Design review of the part built by this model. Coordinates are the model's own, in mm. A direction names the side the tool comes from. Coordinates: 2 decimals unless noted, no trailing zeros. Loops run counter-clockwise (first coordinate to the right, second up) from the corner with the lowest first, then second, coordinate; pieces in that order, holes last. Notation, with made-up numbers: (27, -6.5) -> (52, -6.5) arc R21 cw to (52, 5.5) -> close; hole circle Ø5 at (84, 57). An arc over 180 degrees is marked (long way). Use a Markdown table: item, result. Add a question column.
Q1. For probe 1 along Y at (x, z) = (0, 7); probe 2 along Y at (x, z) = (0, 2); probe 3 along X at (y, z) = (8, 31), list the stretches that pass through material, from the lowest coordinate up.
Q2. Take a section at B-B on y = 5.5. Write out the cut boundary in (x, z) (3 decimals), plus the area to 3 significant figures.
Q3. Clearance check with flat-ended pins moving along their axes: pin 1 Ø0.9 at (x, z) = (-17, 30.5) entering from -Y; pin 2 Ø5 at (x, z) = (3.5, 25) entering from -Y; pin 3 Ø10 at (x, y) = (-5, 1) entering from +Z. State where each tip first meets the part, or that it passes through.
Q4. Take a section at D-D on x = -17. Write out the cut boundary in (y, z) (3 decimals), plus the area to 3 significant figures.
Q5. For faces 1 (the face through (17, -1.016, 27)), 2 (the face through (17, -8.382, 27)), 3 (the face through (-3, -8, 5.398)), list the 3-axis set-ups (+Z, -Z, +X, -X, +Y, -Y) from which the entire face can be reached by the end or side of a thin tool; tool diameter is ignored.
Q6. Draft analysis for pull direction Y (two halves, no side actions). For faces 4 (the face through (15.249, -5, 27)), 5 (the face through (-19.431, 7, 27)), 6 (the face through (-17, -8.382, 27)), state which applies: pulls with the +Y half, pulls with the -Y half, needs draft (parallel to the pull), parting line crosses it, or undercut.
from build123d import *

# Parameters (mm, degrees)
SKETCH1_W                                         = 48.26
SKETCH1_H                                         = 38.1
BOSS_EXTRUDE1_DEPTH                               = 10.16
BOSS_EXTRUDE3_DEPTH                               = 34.925
CBORE_FOR_5_16_SOCKET_HEAD_CAP_SCREW1_D           = 8.2042
CBORE_FOR_5_16_SOCKET_HEAD_CAP_SCREW1_CBORE_D     = 13.49502
CBORE_FOR_5_16_SOCKET_HEAD_CAP_SCREW1_CBORE_DEPTH = 5.3975
SKETCH7_R                                         = 5.715
CUT_EXTRUDE2_DEPTH                                = 1.905
SKETCH8_W                                         = 4.182361547
SKETCH8_H                                         = 7.366
BOSS_EXTRUDE4_DEPTH                               = 34.925
FILLET2_R                                         = 0.635
FILLET3_R                                         = 0.635
FILLET1_R                                         = 0.635


with BuildPart() as part:
    # Sketch1 → Boss-Extrude1 (new body)
    with BuildSketch(Plane.XY):
        Rectangle(SKETCH1_W, SKETCH1_H)
    extrude(amount=BOSS_EXTRUDE1_DEPTH)

    # Sketch5 → Boss-Extrude3 (add)
    with BuildSketch(Plane.XY.offset(10.16)):
        Polygon((-24.13, -19.05), (-24.13, 19.05), (24.13, 19.05), (24.13, -19.05), (19.431, -19.05), (19.431, 14.351), (-19.431, 14.351), (-19.431, -19.05), align=None)
    extrude(amount=BOSS_EXTRUDE3_DEPTH)

    # CBORE for 5/16 Socket Head Cap Screw1 (through all)
    with Locations(Plane(origin=(0, 0, 0), x_dir=(-1, 0, 0), z_dir=(0, 0, -1))):
        with Locations((0, -4.699)):
            CounterBoreHole(CBORE_FOR_5_16_SOCKET_HEAD_CAP_SCREW1_D / 2, CBORE_FOR_5_16_SOCKET_HEAD_CAP_SCREW1_CBORE_D / 2, CBORE_FOR_5_16_SOCKET_HEAD_CAP_SCREW1_CBORE_DEPTH)

    # Sketch7 → Cut-Extrude2 (cut)
    with BuildSketch(Plane.XY.offset(10.16)):
        with Locations((0, -4.699)):
            Circle(SKETCH7_R)
    extrude(amount=-CUT_EXTRUDE2_DEPTH, mode=Mode.SUBTRACT)

    # Sketch8 → Boss-Extrude4 (add)
    with BuildSketch(Plane.XY.offset(10.16)):
        with Locations((-17.339819227, -4.699)):
            Rectangle(SKETCH8_W, SKETCH8_H)
    boss_extrude4 = extrude(amount=BOSS_EXTRUDE4_DEPTH)

    # Fillet2
    fillet2_edges = [part.edges().sort_by_distance(p)[0] for p in [
        (-19.431, 14.351, 27.6225),
        (19.431, 14.351, 27.6225),
    ]]
    fillet(fillet2_edges, radius=FILLET2_R)

    # Fillet3
    fillet3_edges = [part.edges().sort_by_distance(p)[0] for p in [
        (-19.431, -19.05, 27.6225),
        (24.13, -19.05, 22.5425),
        (-24.13, -19.05, 22.5425),
        (-24.13, 19.05, 22.5425),
        (24.13, 19.05, 22.5425),
    ]]
    fillet(fillet3_edges, radius=FILLET3_R)

    # Mirror2: Boss-Extrude4 across plane
    add(boss_extrude4.mirror(Plane(origin=(0, 0, 0), x_dir=(0, 0, 1), z_dir=(1, 0, 0))))

    # Fillet1
    fillet1_edges = [part.edges().sort_by_distance(p)[0] for p in [
        (19.431, -1.016, 27.6225),
        (19.431, -8.382, 27.6225),
        (15.248638453, -8.382, 27.6225),
        (15.248638453, -1.016, 27.6225),
        (-15.248638453, -8.382, 27.6225),
        (-15.248638453, -1.016, 27.6225),
        (-19.431, -1.016, 27.6225),
        (-19.431, -8.382, 27.6225),
    ]]
    fillet(fillet1_edges, radius=FILLET1_R)


solid = part.part
Answer list:
| question | item | result |
|---|---|---|
| 1 | probe 1 | -19.05 to -8.8, -0.6 to 19.05 |
| 1 | probe 2 | -19.05 to -11.45, 2.05 to 19.05 |
| 1 | probe 3 | -24.13 to -19.43, 19.43 to 24.13 |
| 2 | outline | (-24.13, 0) -> (24.13, 0) -> (24.13, 45.085) -> (19.431, 45.085) -> (19.431, 10.16) -> (-19.431, 10.16) -> (-19.431, 45.085) -> (-24.13, 45.085) -> close |
| 2 | area | 819 mm² |
| 3 | pin 1 | y = -8.38 |
| 3 | pin 2 | y = 14.35 |
| 3 | pin 3 | z = 10.16 |
| 4 | outline | (-19.05, 0) -> (19.05, 0) -> (19.05, 45.085) -> (14.351, 45.085) -> (14.351, 10.16) -> (-1.016, 10.16) -> (-1.016, 45.085) -> (-8.382, 45.085) -> (-8.382, 10.16) -> (-19.05, 10.16) -> close |
| 4 | area | 808 mm² |
| 5 | face 1 | +Z |
| 5 | face 2 | +Z, -Y |
| 5 | face 3 | -Z |
| 6 | face 4 | needs draft |
| 6 | face 5 | undercut |
| 6 | face 6 | pulls with the -Y half |
